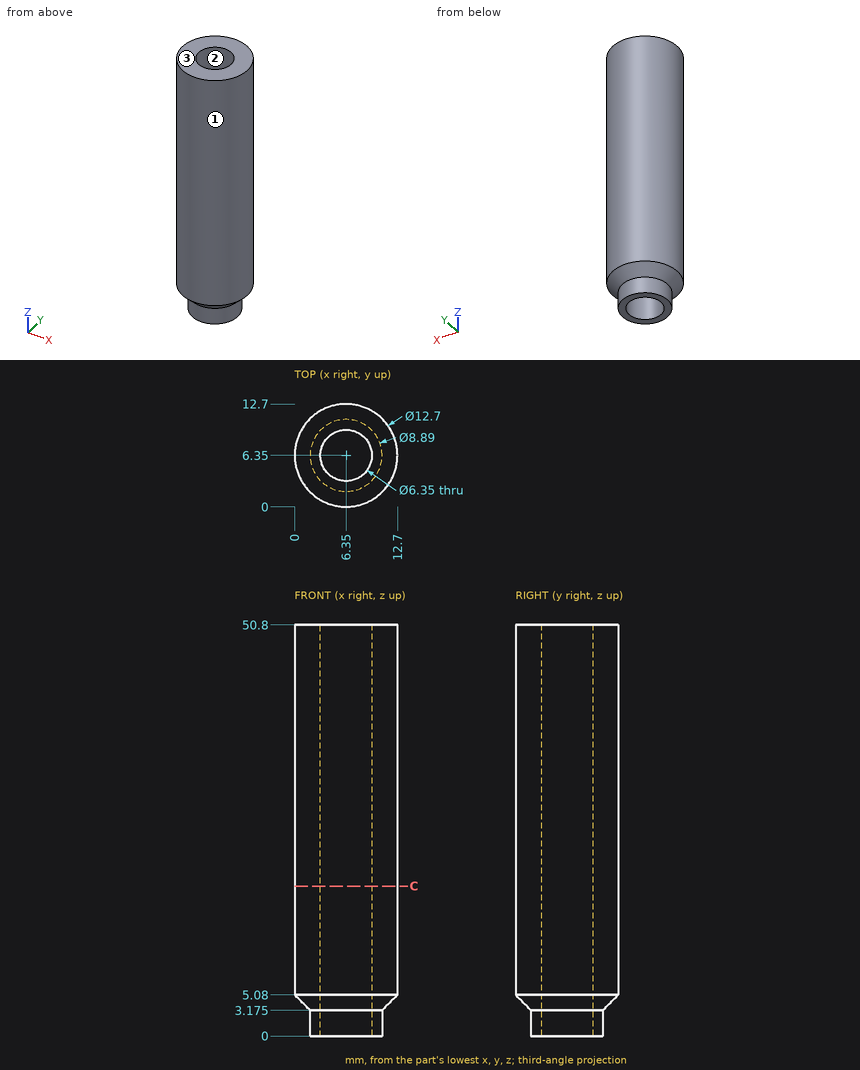
Job drawing, mm, ordinate dimensions from the low corner. One solid piece. Round coordinates to 2 decimals unless told otherwise and drop trailing zeros. Loops run counter-clockwise (first coordinate to the right, second up) from the corner with the lowest first, then second, coordinate; pieces in that order, holes last. Notation, with made-up numbers: M 33,-20.5 L 43,-20.5 A20 ccw 43,14.5 Z; hole C 64.25,25.25 d9. An arc over 180 degrees is marked long. Answer as CSV lines item,"result".
1. Wall check: probe 1 along Y at (x, z) = (6.35, 39.5) (3 decimals); probe 2 along Y at (x, z) = (5.25, 15); probe 3 along X at (y, z) = (4.25, 32). Give the ranges that are in metal, low to high. Write a range as [from, to].
Resolved:
probe 1,"y = [0, 3.175], [9.525, 12.7]"
probe 2,"y = [0.1, 3.37], [9.33, 12.6]"
probe 3,"x = [0.36, 3.97], [8.73, 12.34]"
2. Two-plate mould, pull along Y, no slides. Class the marked faces 1, 2 and 3: released by +Y, released by -Y, zero draft, split by the parting line, or undercut.
Resolved:
face 1,"split by the parting line"
face 2,"undercut"
face 3,"zero draft"
3. Cut at C-C on z = 18.5. Write the cut outline in (x, y) (3 decimals), then the cut area to 3 significant figures.
Resolved:
outline,"C 6.35,6.35 d12.7; hole C 6.35,6.35 d6.35"
area,"95.0 mm²"
4. Flat gauge pins, fed straight in: P1, Ø4, axis at x = 9, z = 8, coming from the -Y side; P2, Ø5.5, axis at x = 6.35, y = 6.35, coming from the -Z side (1 decimal). Where does each tip first touch, or does it go through?
Resolved:
P1,"stops at y = 0.03"
P2,"passes through"
